```python
from build123d import *

# Parameters (mm, degrees)
SKETCH1_R           = 8
SKETCH1_R_2         = 3.7
BOSS_EXTRUDE1_DEPTH = 2
SKETCH2_R           = 5.5
SKETCH2_R_2         = 3.7
BOSS_EXTRUDE2_DEPTH = 4
FILLET2_R           = 0.6
CHAMFER2_SIZE       = 0.2
SKETCH3_R           = 4.1
CUT_EXTRUDE1_DEPTH  = 2.5
CHAMFER3_SIZE2      = 0.4
CHAMFER3_SIZE       = 0.230940108


with BuildPart() as part:
    # Sketch1 → Boss-Extrude1 (new body)
    with BuildSketch(Plane(origin=(0, 0, 0), x_dir=(1, 0, 0), z_dir=(0, 1, 0))):
        with Locations(Location((0, 0, 0), (0, 0, 270))):
            Circle(SKETCH1_R)
        with Locations(Location((0, 0, 0), (0, 0, 270))):
            Circle(SKETCH1_R_2, mode=Mode.SUBTRACT)
    extrude(amount=BOSS_EXTRUDE1_DEPTH)

    # Sketch2 → Boss-Extrude2 (add)
    with BuildSketch(Plane(origin=(0, 2, 0), x_dir=(1, 0, 0), z_dir=(0, 1, 0))):
        with Locations(Location((0, 0, 0), (0, 0, 270))):
            Circle(SKETCH2_R)
        with Locations(Location((0, 0, 0), (0, 0, 270))):
            Circle(SKETCH2_R_2, mode=Mode.SUBTRACT)
    extrude(amount=BOSS_EXTRUDE2_DEPTH)

    # Fillet2
    fillet2_edges = [part.edges().sort_by_distance(p)[0] for p in [
        (0, 2, -5.5),
    ]]
    fillet(fillet2_edges, radius=FILLET2_R)

    # Chamfer2
    chamfer2_edges = [part.edges().sort_by_distance(p)[0] for p in [
        (0, 6, -3.7),
    ]]
    chamfer(chamfer2_edges, length=CHAMFER2_SIZE)

    # Sketch3 → Cut-Extrude1 (cut)
    with BuildSketch(Plane.XZ):
        with Locations(Location((0, 0, 0), (0, 0, 270))):
            Circle(SKETCH3_R)
    extrude(amount=-CUT_EXTRUDE1_DEPTH, mode=Mode.SUBTRACT)

    # Chamfer3
    chamfer3_edges = [part.edges().sort_by_distance(p)[0] for p in [
        (0, 2.5, -3.7),
    ]]
    chamfer3_side = [part.faces().sort_by_distance(p)[0] for p in [
        (0, 2.504618802, -3.7),
    ]]
    chamfer(chamfer3_edges, length=CHAMFER3_SIZE - 0.0001, length2=CHAMFER3_SIZE2 - 0.0001, reference=chamfer3_side[0])  # a hair under: the kernel refuses the full size


solid = part.part
```
Check sheet for the modelled part. Datum: model origin and axes. Units: mm. A direction names the side the tool comes from. Round coordinates to 2 decimals unless told otherwise and drop trailing zeros. Loops run counter-clockwise (first coordinate to the right, second up) from the corner with the lowest first, then second, coordinate; pieces in that order, holes last. Notation, with made-up numbers: (57.25, 48) -> (81.25, 48) arc R28 ccw to (81.25, 68) -> close; hole circle Ø8 at (6, 61). An arc over 180 degrees is marked (long way). Write item = value, one per line. Start each with the question number.
1) Release check for a two-part mould opening along Z. For faces 1 (the flat face through (2, 0, -4)), 2 (the cylindrical face through (-5.37, 4.28, -1.19)), 3 (the cylindrical face through (4.065, 1.232, 0.534)) record: released by +Z, released by -Z, zero draft, split by the parting line, or undercut.
2) Thickness scan on probe 1 along X at (y, z) = (4.7, 0); probe 2 along X at (y, z) = (1.3, 0); probe 3 along Z at (x, y) = (-2.25, 1.95). Record the ranges inside material, lowest first.
3) Sectioned sample at C-C, the plane y = 4.7. Record the cut outline in (x, z).
4) Set-up check for faces 4 (the cylindrical face through (-7.81, 0.99, -1.73)), 5 (the flat face through (-6, 2, -2)): record each of +Z, -Z, +X, -X, +Y, -Y from which the full face is reachable in a straight line by a thin tool's end or side.
5) Gauge pin test, flat ends, axial feed: pin 1 Ø1 at (x, y) = (4.5, 5) entering from -Z; pin 2 Ø4.5 at (x, z) = (0, 0) entering from +Y; pin 3 Ø1.5 at (x, y) = (3.5, 4.5) entering from -Z; pin 4 Ø1 at (y, z) = (1.5, 5) entering from +X. Record the tip position at first contact, or that the pin passes through.
6) Sectioned sample at D-D, the plane x = -6.5. Record the cut outline in (y, z), plus the area to 3 significant figures.
Results are:
q1.face_1 = zero draft
q1.face_2 = split by the parting line
q1.face_3 = undercut
q2.probe_1 = -5.5 to -3.7, 3.7 to 5.5
q2.probe_2 = -8 to -4.1, 4.1 to 8
q2.probe_3 = -7.68 to -3.43, 3.43 to 7.68
q3.outline = circle Ø11 at (0, 0); hole circle Ø7.4 at (0, 0)
q4.face_4 = +Y, -Y
q4.face_5 = +Y
q5.pin_1 = -3.77
q5.pin_2 = through
q5.pin_3 = -4.76
q5.pin_4 = 6.61
q6.outline = (0, -4.66) -> (2, -4.66) -> (2, 4.66) -> (0, 4.66) -> close
q6.area = 18.7 mm^2
